from build123d import *

# Parameters (mm, degrees)
SKETCH1_W                = 200
SKETCH1_H                = 41
BOSS_EXTRUDE1_DEPTH      = 20
FILLET1_R                = 5
SKETCH4_R                = 2.5
CUT_EXTRUDE1_DEPTH       = 206.136539895
SKETCH5_W                = 190
SKETCH5_H                = 31
CUT_EXTRUDE2_DEPTH       = 15
M4_CLEARANCE_HOLE1_D     = 4.5
M4_CLEARANCE_HOLE1_DEPTH = 8
M4_CLEARANCE_HOLE1_TIP   = 1.351936393
CUT_EXTRUDE3_START       = -3.5
CUT_EXTRUDE3_DEPTH       = 7.5
LPATTERN1_COUNT          = 2
LPATTERN1_PITCH          = 70
LPATTERN1_COUNT_DIR2     = 2
LPATTERN1_PITCH_DIR2     = 26


with BuildPart() as part:
    # Sketch1 → Boss-Extrude1 (new body)
    with BuildSketch(Plane(origin=(0, 0, 0), x_dir=(1, 0, 0), z_dir=(0, 1, 0))):
        with Locations((100, 20.5)):
            Rectangle(SKETCH1_W, SKETCH1_H)
    extrude(amount=BOSS_EXTRUDE1_DEPTH)

    # Fillet1
    fillet1_edges = [part.edges().sort_by_distance(p)[0] for p in [
        (0, 10, -41),
        (200, 10, -41),
        (200, 10, 0),
        (0, 10, 0),
    ]]
    fillet(fillet1_edges, radius=FILLET1_R)

    # Sketch4 → Cut-Extrude1 (cut, through all)
    with BuildSketch(Plane.ZY):
        with Locations((-20.5, 8)):
            Circle(SKETCH4_R)
    extrude(amount=-CUT_EXTRUDE1_DEPTH, mode=Mode.SUBTRACT)

    # Sketch5 → Cut-Extrude2 (cut)
    with BuildSketch(Plane.XZ):
        with Locations((100, -20.5)):
            Rectangle(SKETCH5_W, SKETCH5_H)
    extrude(amount=-CUT_EXTRUDE2_DEPTH, mode=Mode.SUBTRACT)

    # M4 Clearance Hole1
    with Locations(Plane(origin=(135, 20, -7.5), x_dir=(0, 0, 1), z_dir=(0, 1, 0))):
        with Locations((0, 0), (-26, -70), (-26, 0), (0, -70)):
            Hole(M4_CLEARANCE_HOLE1_D / 2, depth=M4_CLEARANCE_HOLE1_DEPTH)
            with Locations((0, 0, -(M4_CLEARANCE_HOLE1_DEPTH + M4_CLEARANCE_HOLE1_TIP / 2))):  # 118° drill point
                Cone(0, M4_CLEARANCE_HOLE1_D / 2, M4_CLEARANCE_HOLE1_TIP, mode=Mode.SUBTRACT)

    # Sketch7 → Cut-Extrude3 (cut)
    with BuildSketch(Plane.XZ.offset(-15).offset(CUT_EXTRUDE3_START)):
        Polygon((65, -12.407477288), (69.25, -9.953738644), (69.25, -5.046261356), (65, -2.592522712), (60.75, -5.046261356), (60.75, -9.953738644), align=None)
    cut_extrude3 = extrude(amount=CUT_EXTRUDE3_DEPTH, mode=Mode.SUBTRACT)

    # LPattern1: Cut-Extrude3 2 × 2
    with Locations(*[(i * LPATTERN1_PITCH, 0, -j * LPATTERN1_PITCH_DIR2) for i in range(LPATTERN1_COUNT) for j in range(LPATTERN1_COUNT_DIR2) if (i, j) != (0, 0)]):
        add(cut_extrude3, mode=Mode.SUBTRACT)


solid = part.part
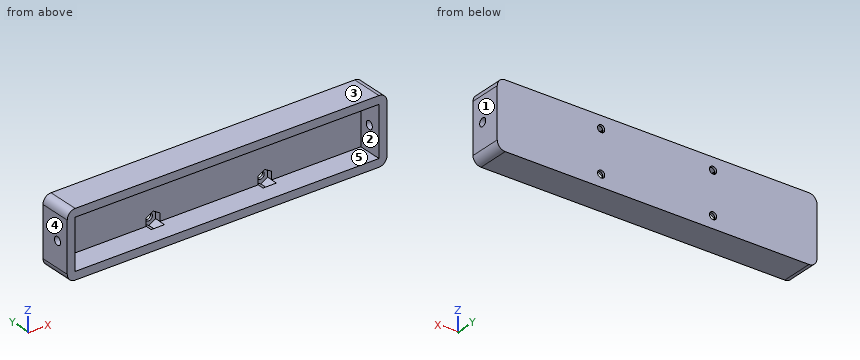
Source: CAD feature listing. Evaluate the final solid. Frame: model axes, mm. Face numbers are marked on the shaded views. A direction names the side the tool comes from. Give positions to 0.01 mm unless a question says otherwise; leave off trailing zeros. Order: outer loops, then holes, each group sorted by start corner. A loop starts at its lowest first (then second) coordinate and runs counter-clockwise, first axis right, second up. Notation, with made-up numbers: (30, 41) -> (79, 41) arc R34 cw to (79, 75) -> close; hole circle Ø2 at (-21, 80.25). An arc over 180 degrees is marked (long way). Use a Markdown table: item, result.
1) Section query B-B, the plane y = 2. Return the cut outline in (x, z), then the cut area to 3 significant figures.
Answer list:
| item | result |
|---|---|
| outline | (0, -36) arc R5 ccw to (5, -41) -> (195, -41) arc R5 ccw to (200, -36) -> (200, -5) arc R5 ccw to (195, 0) -> (5, 0) arc R5 ccw to (0, -5) -> close; hole (5, -36) -> (195, -36) -> (195, -5) -> (5, -5) -> close |
| area | 2,290 mm² |
2) Ray query, line 1 along Z through (x, y) = (135, 19.7); line 2 along X through (y, z) = (19.35, -7.5); line 3 along X through (y, z) = (17.5, -5.5). Return the intervals inside material, ascending. Write a range as [from, to].
Answer list:
| item | result |
|---|---|
| line 1 | [-41, -35.75], [-31.25, -9.75], [-5.25, 0] |
| line 2 | [0, 62.75], [67.25, 132.75], [137.25, 200] |
| line 3 | [0, 60.75], [69.25, 130.75], [139.25, 200] |
3) Section query C-C, the plane x = 48.5. Return the cut outline in (y, z).
Answer list:
| item | result |
|---|---|
| outline | (0, -41) -> (20, -41) -> (20, 0) -> (0, 0) -> (0, -5) -> (15, -5) -> (15, -36) -> (0, -36) -> close |
4) Section query D-D, the plane z = -20.5. Return the cut outline in (x, y), then the cut area to 3 significant figures.
Answer list:
| item | result |
|---|---|
| outline | (0, 0) -> (5, 0) -> (5, 5.5) -> (0, 5.5) -> close; (0, 10.5) -> (5, 10.5) -> (5, 15) -> (195, 15) -> (195, 10.5) -> (200, 10.5) -> (200, 20) -> (0, 20) -> close; (195, 0) -> (200, 0) -> (200, 5.5) -> (195, 5.5) -> close |
| area | 1,100 mm² |
5) Reachability of the marked faces 4 and 5 from +Z, -Z, +X, -X, +Y, -Y: full face, straight path, thin tool, end or side. Return the list, or none.
Answer list:
| item | result |
|---|---|
| face 4 | +Z, -Z, -X, +Y, -Y |
| face 5 | -Y |
6) Section query A-A, the plane z = -33.5. Return the cut outline in (x, y), then the cut area to 3 significant figures.
Answer list:
| item | result |
|---|---|
| outline | (0, 0) -> (5, 0) -> (5, 15) -> (60.75, 15) -> (60.75, 18.5) -> (62.75, 18.5) -> (62.75, 20) -> (0, 20) -> close; (67.25, 18.5) -> (69.25, 18.5) -> (69.25, 15) -> (130.75, 15) -> (130.75, 18.5) -> (132.75, 18.5) -> (132.75, 20) -> (67.25, 20) -> close; (137.25, 18.5) -> (139.25, 18.5) -> (139.25, 15) -> (195, 15) -> (195, 0) -> (200, 0) -> (200, 20) -> (137.25, 20) -> close |
| area | 1,080 mm² |
7) Mould query, pull axis X, two halves, no side actions, for the marked faces 1, 2 and 3. Classes: +X half, -X half, draft (parallel to the pull), parting line (faces both ways), or undercut.
Answer list:
| item | result |
|---|---|
| face 1 | +X half |
| face 2 | undercut |
| face 3 | draft |
8) Contact query for flat-ended pins moving along their axis: P1, Ø2.5, axis at x = 63, z = -32.5, coming from the -Y side; P2, Ø15.5, axis at x = 127, z = -21, coming from the -Y side; P3, Ø3, axis at y = 8, z = -20.5, coming from the -X side. Output: stop coordinate, or through.
Answer list:
| item | result |
|---|---|
| P1 | y = 18.5 |
| P2 | y = 15 |
| P3 | through |
